Autodesk Inventor part; units mm, degrees
ref_plane "YZ Plane" through (0, 0, 0) normal (1, 0, 0) x (0, 1, 0)
ref_plane "XZ Plane" through (0, 0, 0) normal (0, 1, 0) x (-1, 0, 0)
ref_plane "XY Plane" through (0, 0, 0) normal (0, 0, 1) x (1, 0, 0)
sketch "Sketch1" plane through (0, 0, 0) normal (0, 1, 0) x (-1, 0, 0)
  circle A0 centre (0, 0) radius 2.5
  dimension "d0" = 5
extrude "Extrusion1" add sketch "Sketch1" along normal blind 72
sketch "Sketch2" plane through (0, 72, 0) normal (0, 1, 0) x (1, 0, 0)
  circle A0 centre (0, 0) radius 2.5
  line L0 (-2, -1.5) -> (-2, 1.5)
  dimension "d3" = 2
extrude "Extrusion2" cut sketch "Sketch2" against normal blind 15 contours L0 A0 picked at (-2.0912, -0.3466)
chamfer "Chamfer1" distance 0.2 angle 45 1 edges at (2.5, 72, 0)
chamfer "Chamfer2" distance 0.2 angle 45 1 edges at (2.5, 0, 0)
properties part number "Stepper Shaft"
Here's how the part is built. I have some questions about the finished solid (model axes, mm). Give positions to 0.01 mm unless a question says otherwise; leave off trailing zeros. Loops run counter-clockwise (first coordinate to the right, second up) from the corner with the lowest first, then second, coordinate; pieces in that order, holes last. Notation, with made-up numbers: (85.5, 5) -> (129.5, 5) arc R27 ccw to (129.5, 37) -> close; hole circle Ø11 at (14.5, 4.25). An arc over 180 degrees is marked (long way). One line per item, written item: value.
Q1. Suppose I cut it at B-B on y = 48. Please give me the cut outline in (x, z), then the cut area to 3 significant figures.
Answers follow:
outline: circle Ø5 at (0, 0)
area: 19.6 mm^2
Q2. We'd pull the mould along Y, two halves only. Please class faces 1 (the face through (2.5, 35.5, -0.1)), 2 (the face through (0, 0, 0)), 3 (the face through (0, 72, 0)): pulls with the +Y half, pulls with the -Y half, needs draft (parallel to the pull), parting line crosses it, or undercut.
Answers follow:
face 1: needs draft
face 2: pulls with the -Y half
face 3: pulls with the +Y half
Q3. I'm going to push flat-ended pins straight in: pin 1 Ø1.5 at (y, z) = (66, -0.5) entering from -X; pin 2 Ø1.5 at (y, z) = (55.5, 2) entering from -X. Where does each tip first touch, or does it pass through?
Answers follow:
pin 1: x = -2
pin 2: x = -2.17
Q4. If I drill on line 1 along X through (y, z) = (12.5, 0.15); line 2 along X through (y, z) = (68, 0.25); line 3 along Z through (x, y) = (-1, 41.5), over which ranges is the centre line in solid material (lowest first)?
Answers follow:
line 1: -2.5 to 2.5
line 2: -2 to 2.49
line 3: -2.29 to 2.29
Q5. Suppose I cut it at A-A on z = 0. Please give me the cut outline in (x, y), then the cut area to 3 significant figures.
Answers follow:
outline: (-2.5, 0.2) -> (-2.3, 0) -> (2.3, 0) -> (2.5, 0.2) -> (2.5, 71.8) -> (2.3, 72) -> (-2, 72) -> (-2, 57) -> (-2.5, 57) -> close
area: 352 mm^2
